Build history of the part. All positions in model axes, mm. A direction names the side the tool comes from. Give positions to 0.01 mm unless a question says otherwise; leave off trailing zeros. Loops run counter-clockwise (first coordinate to the right, second up) from the corner with the lowest first, then second, coordinate; pieces in that order, holes last. Notation, with made-up numbers: (44.5, 78.5) -> (87.5, 78.5) arc R26 ccw to (87.5, 109.5) -> close; hole circle Ø7 at (56.25, -29). An arc over 180 degrees is marked (long way). Answer as a JSON object with one key per item and string values. Group by question number.
Q1. Band-saw the part on C-C, the plane x = 147. Write the cut outline in (y, z).
Q2. Drop flat-ended pins along their axis: pin 1 (2.5 mm diameter, centred on x = 99, y = 2, fed in from -Z); pin 2 (2.5 mm diameter, centred on y = 3, z = -146, fed in from +X); pin 3 (1 mm diameter, centred on y = 4, z = -41, fed in from +X). Give the stop position or say it passes through.
Q3. Band-saw the part on A-A, the plane y = 3.5. Write the cut outline in (x, z), plus the area to 3 significant figures.
Q4. Two-plate mould, pull along X, no slides. Class faces 1 (the flat face through (157, 2, -8.188)), 2 (the flat face through (25.4, 2, -101)), 3 (the flat face through (22, 2, -152.4)): pulls with the +X half, pulls with the -X half, needs draft (parallel to the pull), parting line crosses it, or undercut.
Q5. Band-saw the part on B-B, the plane z = -139.7. Write the cut outline in (x, y), plus the area to 3 significant figures.
Q6. Wall check: probe 1 along X at (y, z) = (2, -139.7); probe 2 along Z at (x, y) = (156.5, 4.25); probe 3 along Z at (x, y) = (121, 1.45). Give the ranges that are in metal, low to high. Write a range as from..to.
Q7. Tool access for faces 4 (the flat face through (158, 2, -17.212)), 5 (the flat face through (88, 2, 0)), 6 (the flat face through (102, 2, -25.4)): list every direction of +Z, -Z, +X, -X, +Y, -Y with a clear straight run to the whole face (end or side of a thin tool).
Q8. Band-saw the part on D-D, the plane z = -48. Write the cut outline in (x, y).
from build123d import *

# Parameters (mm, degrees)
BOSS_EXTRUDE1_DEPTH = 4.7625
SKETCH2_R           = 1
CUT_EXTRUDE1_DEPTH  = 8.89


with BuildPart() as part:
    # Sketch1 → Boss-Extrude1 (new body)
    with BuildSketch(Plane(origin=(0, 0, 0), x_dir=(1, 0, 0), z_dir=(0, 1, 0))):
        with BuildLine():
            Line((25.4, 0), (152.4, 0))
            Line((152.4, 0), (152.4, 7.1875))
            ThreePointArc((152.4, 7.1875), (152.692893219, 7.894606781), (153.4, 8.1875))
            Line((153.4, 8.1875), (161.495448411, 8.1875))
            ThreePointArc((161.495448411, 8.1875), (171.7, 12.7), (161.495448411, 17.2125))
            Line((161.495448411, 17.2125), (153.4, 17.2125))
            ThreePointArc((153.4, 17.2125), (152.692893219, 17.505393219), (152.4, 18.2125))
            Line((152.4, 18.2125), (152.4, 25.4))
            Line((152.4, 25.4), (50.8, 25.4))
            ThreePointArc((50.8, 25.4), (32.839487758, 32.839487758), (25.4, 50.8))
            Line((25.4, 50.8), (25.4, 152.4))
            Line((25.4, 152.4), (18.4625, 152.4))
            ThreePointArc((18.4625, 152.4), (17.755393219, 152.107106781), (17.4625, 151.4))
            Line((17.4625, 151.4), (17.4625, 143.900130206))
            ThreePointArc((17.4625, 143.900130206), (12.7, 133.35), (7.9375, 143.900130206))
            Line((7.9375, 143.900130206), (7.9375, 151.4))
            ThreePointArc((7.9375, 151.4), (7.644606781, 152.107106781), (6.9375, 152.4))
            Line((6.9375, 152.4), (0, 152.4))
            Line((0, 152.4), (0, 25.4))
            ThreePointArc((0, 25.4), (7.439487758, 7.439487758), (25.4, 0))
        make_face()
    extrude(amount=BOSS_EXTRUDE1_DEPTH)

    # Sketch2 → Cut-Extrude1 (cut)
    with BuildSketch(Plane(origin=(0, 4.7625, 0), x_dir=(1, 0, 0), z_dir=(0, 1, 0))):
        with Locations(Location((19.05, 19.05, 0), (0, 0, 270))):
            Circle(SKETCH2_R)
    extrude(amount=-CUT_EXTRUDE1_DEPTH, mode=Mode.SUBTRACT)


solid = part.part
Worked answers:
{
 "1": {"outline": "(0, -25.4) -> (4.76, -25.4) -> (4.76, 0) -> (0, 0) -> close"},
 "2": {"pin 1": "z = -25.4", "pin 2": "x = 25.4", "pin 3": "x = 27.58"},
 "3": {"outline": "(0, -152.4) -> (6.94, -152.4) arc R1 ccw to (7.94, -151.4) -> (7.94, -143.9) arc R6.35 cw (long way) to (17.46, -143.9) -> (17.46, -151.4) arc R1 ccw to (18.46, -152.4) -> (25.4, -152.4) -> (25.4, -50.8) arc R25.4 cw to (50.8, -25.4) -> (152.4, -25.4) -> (152.4, -18.21) arc R1 cw to (153.4, -17.21) -> (161.5, -17.21) arc R6.1 ccw (long way) to (161.5, -8.19) -> (153.4, -8.19) arc R1 cw to (152.4, -7.19) -> (152.4, 0) -> (25.4, 0) arc R25.4 ccw to (0, -25.4) -> close; hole circle Ø2 at (19.05, -19.05)", "area": "7,090 mm2"},
 "4": {"face 1": "undercut", "face 2": "pulls with the +X half", "face 3": "needs draft"},
 "5": {"outline": "(0, 0) -> (6.35, 0) -> (6.35, 4.76) -> (0, 4.76) -> close; (19.05, 0) -> (25.4, 0) -> (25.4, 4.76) -> (19.05, 4.76) -> close", "area": "60.5 mm2"},
 "6": {"probe 1": "0..6.35, 19.05..25.4", "probe 2": "-17.21..-8.19", "probe 3": "-25.4..0"},
 "7": {"face 4": "-Z, +Y, -Y", "face 5": "+Z, +X, -X, +Y, -Y", "face 6": "-Z, +X, +Y, -Y"},
 "8": {"outline": "(0, 0) -> (25.55, 0) -> (25.55, 4.76) -> (0, 4.76) -> close"}
}
